The figure shows three views and two pictorial views of one solid part (mm, origin at its lowest corner). Answer the questions. A direction names the side the tool comes from. Coordinates: 2 decimals unless noted, no trailing zeros. Order: outer loops, then holes, each group sorted by start corner. A loop starts at its lowest first (then second) coordinate and runs counter-clockwise, first axis right, second up. Notation, with made-up numbers: (49.25, -7.5) - (57.25, -7.5) arc R30 cw to (57.25, 29.5) - close; hole circle Ø10 at (71.5, 9.25). An arc over 180 degrees is marked (long way). Use one line per item in the form item = value.
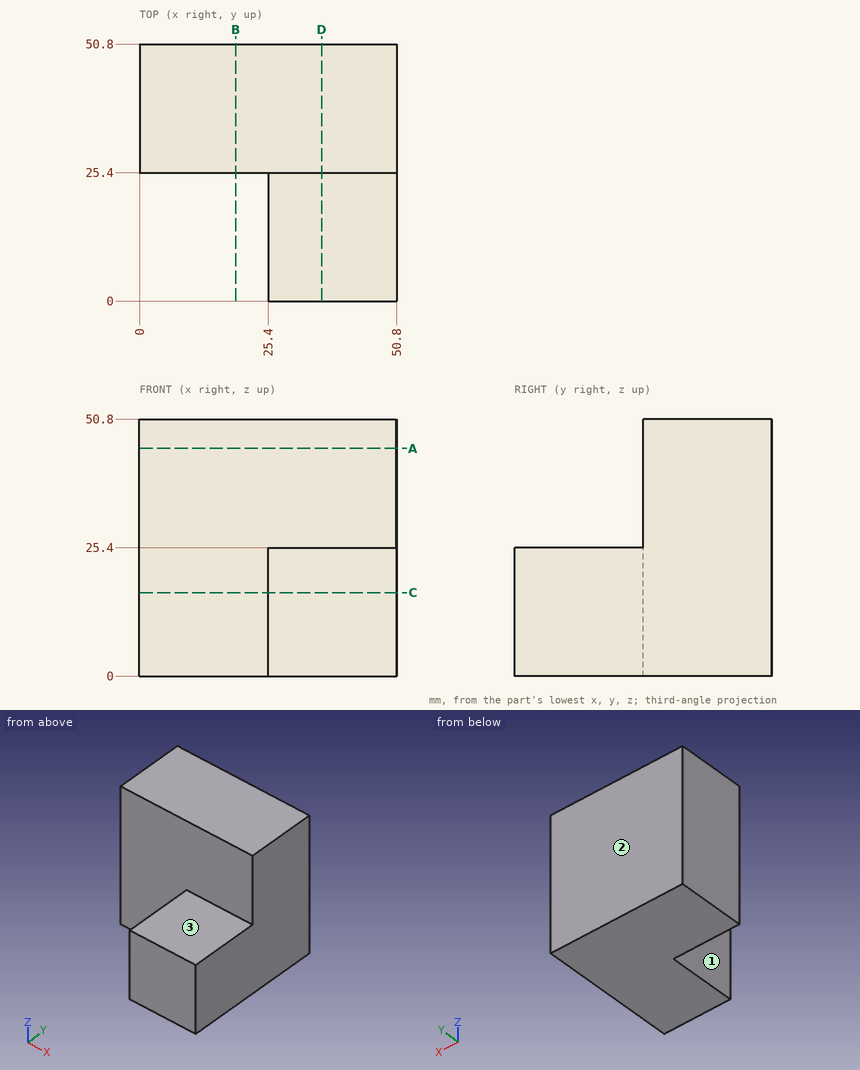
(1) Which of the six approach directions +Z, -Z, +X, -X, +Y, -Y give full straight-line access (tool end or side, diameter ignored) to the marked faces 1, 2 and 3?
Answer list:
face_1 = +Z, -Z, -X, -Y
face_2 = +Z, -Z, +X, -X, +Y
face_3 = +Z, +X, -X, -Y
(2) Section B-B, the plane x = 19 is taken. Write down the section's boundary in (y, z), then the cut area to 3 significant figures.
Answer list:
outline = (25.4, 0) - (50.8, 0) - (50.8, 50.8) - (25.4, 50.8) - close
area = 1,290 mm2
(3) Given pin 1 Ø20.5 at (y, z) = (13, 7.5) entering from -X; pin 2 Ø4 at (x, z) = (18.5, 25.5) entering from -Y, each flat-ended and moving along its own axis, determine where each tip first touches the part or whether it passes through.
Answer list:
pin_1 = 25.4
pin_2 = 25.4
(4) Section D-D, the plane x = 36 is taken. Write down the section's boundary in (y, z), then the cut area to 3 significant figures.
Answer list:
outline = (0, 0) - (50.8, 0) - (50.8, 50.8) - (25.4, 50.8) - (25.4, 25.4) - (0, 25.4) - close
area = 1,940 mm2
(5) Straight lines are drawn through the part: L1, parallel to Y at x = 35, z = 41.5; L2, parallel to Z at x = 31.5, y = 11. For each, find the intervals that lie inside material, in ascending order.
Answer list:
L1 = 25.4 to 50.8
L2 = 0 to 25.4
(6) Section C-C, the plane z = 16.5 is taken. Write down the section's boundary in (x, y), then the cut area to 3 significant figures.
Answer list:
outline = (0, 25.4) - (25.4, 25.4) - (25.4, 0) - (50.8, 0) - (50.8, 50.8) - (0, 50.8) - close
area = 1,940 mm2
(7) Section A-A, the plane z = 45 is taken. Write down the section's boundary in (x, y).
Answer list:
outline = (0, 25.4) - (50.8, 25.4) - (50.8, 50.8) - (0, 50.8) - close
